Could you check a few things on this model? Use its own coordinates, in mm. Face numbers are marked on the shaded views. A direction names the side the tool comes from. Give positions to 0.01 mm unless a question says otherwise; leave off trailing zeros. Write each loop counter-clockwise with the first axis right and the second up, starting at its lowest first coordinate (ties: lowest second). Pieces come first, ordered by that corner, then holes. Notation, with made-up numbers: (74, 79.25) - (132, 79.25) arc R12 cw to (132, 99.25) - close; hole circle Ø10 at (1.5, 11). An arc over 180 degrees is marked (long way). Use one line per item in the form item = value.
```python
from build123d import *

# Parameters (mm, degrees)
BOSS_EXTRUDE1_DEPTH = 42
SKETCH4_R           = 6
CUT_EXTRUDE1_DEPTH  = 42
SKETCH6_W           = 14
SKETCH6_H           = 42
BOSS_EXTRUDE2_DEPTH = 42
FILLET1_R           = 21
SKETCH7_R           = 10
CUT_EXTRUDE2_DEPTH  = 42
FILLET4_R           = 5


with BuildPart() as part:
    # Sketch1 → Boss-Extrude1 (new body)
    with BuildSketch(Plane.XY):
        Polygon((0, 0), (-14, 0), (-14, 20), (84, 20), (84, 0), (70, 0), (70, 6), (0, 6), align=None)
    extrude(amount=-BOSS_EXTRUDE1_DEPTH)

    # Sketch4 → Cut-Extrude1 (cut)
    with BuildSketch(Plane(origin=(0, 20, 0), x_dir=(1, 0, 0), z_dir=(0, 1, 0))):
        with Locations(Location((60, 21, 0), (0, 0, 270))):
            Circle(SKETCH4_R)
        with Locations(Location((10, 21, 0), (0, 0, 270))):
            Circle(SKETCH4_R)
    extrude(amount=-CUT_EXTRUDE1_DEPTH, mode=Mode.SUBTRACT)

    # Sketch6 → Boss-Extrude2 (add)
    with BuildSketch(Plane(origin=(0, 20, 0), x_dir=(1, 0, 0), z_dir=(0, 1, 0))):
        with Locations((35, 21)):
            Rectangle(SKETCH6_W, SKETCH6_H)
    extrude(amount=BOSS_EXTRUDE2_DEPTH)

    # Fillet1
    fillet1_edges = [part.edges().sort_by_distance(p)[0] for p in [
        (35, 62, -42),
        (35, 62, 0),
    ]]
    fillet(fillet1_edges, radius=FILLET1_R - 0.0001)  # a hair under: the kernel refuses the full size

    # Sketch7 → Cut-Extrude2 (cut)
    with BuildSketch(Plane(origin=(42, 0, 0), x_dir=(0, 0, -1), z_dir=(1, 0, 0))):
        with Locations((21, 41)):
            Circle(SKETCH7_R)
    extrude(amount=-CUT_EXTRUDE2_DEPTH, mode=Mode.SUBTRACT)

    # Fillet4
    fillet4_edges = [part.edges().sort_by_distance(p)[0] for p in [
        (-14, 20, -21),
        (84, 20, -21),
    ]]
    fillet(fillet4_edges, radius=FILLET4_R)


solid = part.part
```
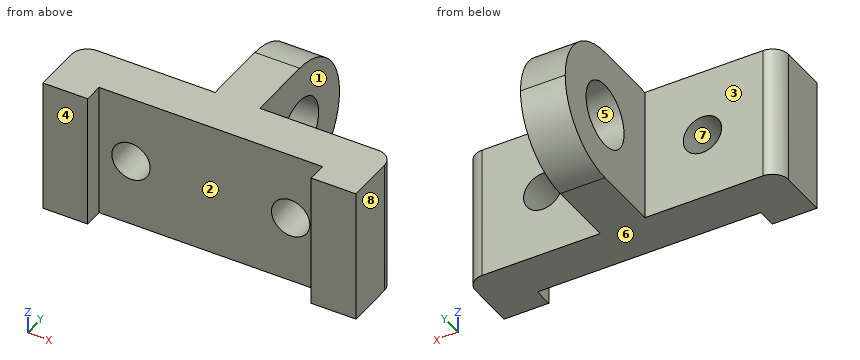
1. For pin 1 (6 mm diameter, centred on y = 55, z = -21.5, fed in from +X); pin 2 (12.5 mm diameter, centred on y = 36.5, z = -23, fed in from -X); pin 3 (1.5 mm diameter, centred on x = 47, z = -14.5, fed in from -Y); pin 4 (2 mm diameter, centred on x = 69.5, z = -28.5, fed in from -Y), each with a flat end and sliding along its axis, tell me the tip position at first contact or that it passes through.
Response values:
pin_1 = 42
pin_2 = 28
pin_3 = 6
pin_4 = 0
2. Imagine slicing it at C-C, the plane y = 47. List the corners of the cut face in (x, z) for me, and give its area (3 significant figures).
Response values:
outline = (28, -41.12) - (42, -41.12) - (42, -29) - (28, -29) - close; (28, -13) - (42, -13) - (42, -0.88) - (28, -0.88) - close
area = 339 mm²
3. If we mould it in two halves opening along Z, with no side actions, what happens to the marked faces 6, 7 and 8? For each: pulls with the +Z half, pulls with the -Z half, needs draft (parallel to the pull), parting line crosses it, or undercut.
Response values:
face_6 = pulls with the -Z half
face_7 = undercut
face_8 = needs draft
4. Imagine slicing it at A-A, the plane x = 60. List the corners of the cut face in (y, z) for me.
Response values:
outline = (6, -42) - (20, -42) - (20, -27) - (6, -27) - close; (6, -15) - (20, -15) - (20, 0) - (6, 0) - close
5. Which directions (+Z, -Z, +X, -X, +Y, -Y) give clear straight access to the entire face, cutting with the end or side of a thin tool? Please do the marked faces 1, 2, 3, 4 and 5.
Response values:
face_1 = +Z, -Z, +X, +Y
face_2 = +Z, -Z, -Y
face_3 = +Z, -Z, -X, +Y
face_4 = +Z, -Z, +X, -X, -Y
face_5 = +X, -X
6. Imagine slicing it at B-B, the plane z = -16. List the corners of the cut face in (x, y) for me, and give its area (3 significant figures).
Response values:
outline = (-14, 0) - (0, 0) - (0, 6) - (6.68, 6) - (6.68, 20) - (-9, 20) arc R5 ccw to (-14, 15) - close; (13.32, 6) - (56.68, 6) - (56.68, 20) - (42, 20) - (42, 32.34) - (28, 32.34) - (28, 20) - (13.32, 20) - close; (28, 49.66) - (42, 49.66) - (42, 61.4) - (28, 61.4) - close; (63.32, 6) - (70, 6) - (70, 0) - (84, 0) - (84, 15) arc R5 ccw to (79, 20) - (63.32, 20) - close
area = 1,680 mm²
7. If I drill on line 1 (X direction, y = 11.5, z = -21); line 2 (X direction, y = 59, z = -16); line 3 (Y direction, x = 39.25, z = -21), over which ranges is the centre line in solid material (lowest first)? Write a range as from..to.
Response values:
line_1 = -14..4, 16..54, 66..84
line_2 = 28..42
line_3 = 6..31, 51..62
